Could you check a few things on this model? Use its own coordinates, in mm. A direction names the side the tool comes from. Round coordinates to 2 decimals unless told otherwise and drop trailing zeros. Write each loop counter-clockwise with the first axis right and the second up, starting at its lowest first coordinate (ties: lowest second). Pieces come first, ordered by that corner, then holes. Notation, with made-up numbers: (-17, 20) -> (24, 20) arc R31 ccw to (24, 49) -> close; hole circle Ø7 at (40.5, 59.25). An arc over 180 degrees is marked (long way). One line per question, with ' | ' between items. Start each with the question number.
1. If I drill on line 1 along Z through (x, y) = (-2.5, -3.5); line 2 along Z through (x, y) = (5, 1); line 3 along X through (y, z) = (-3.25, 11), over which ranges is the centre line in solid material (lowest first)? Write a range as [from, to].
2. For pin 1 Ø2 at (x, z) = (-4, 10.5) entering from +Y; pin 2 Ø2 at (x, z) = (5, 4.5) entering from +Y; pin 3 Ø2 at (y, z) = (-3, 8) entering from -X, each with a flat end and sliding along its axis, tell me the tip position at first contact or that it passes through.
3. For faces 1 (the flat face through (0, 0, 0)), 2 (the conical face through (-0.86, -3.87, 6.76)), which set-ups out of +Z, -Z, +X, -X, +Y, -Y let a thin tool reach every point of the face, with its end or its side?
4. Imagine slicing it at D-D, the plane z = 4.5. List the corners of the cut face in (x, y) for me.
5. Imagine slicing it at C-C, the plane z = 2. List the corners of the cut face in (x, y) for me.
Autodesk Inventor part; units mm, degrees
ref_plane "YZ Plane" through (0, 0, 0) normal (1, 0, 0) x (0, 1, 0)
ref_plane "XZ Plane" through (0, 0, 0) normal (0, 1, 0) x (-1, 0, 0)
ref_plane "XY Plane" through (0, 0, 0) normal (0, 0, 1) x (1, 0, 0)
sketch "Sketch1" plane through (0, 0, 0) normal (0, 0, 1) x (1, 0, 0)
  circle A0 centre (0, 0) radius 6.35
  dimension "d0" = 12.7
extrude "Extrusion1" add sketch "Sketch1" along normal blind 6.604
chamfer "Chamfer1" distance 2.54 angle 45 1 edges at (-6.35, 0, 6.604)
sketch "Sketch2" plane through (0, 0, 6.604) normal (0, 0, 1) x (1, 0, 0)
  circle A0 centre (0, 0) radius 6.35
  dimension "d6" = 12.7
extrude "Extrusion2" add sketch "Sketch2" along normal blind 6.604
chamfer "Chamfer2" distance 2.54 angle 45 1 edges at (-6.35, 0, 6.604)
properties part number "LiftPully" material "Aluminum 6061"
Geometry results:
1) line 1: z = [0, 6.11], [7.09, 13.21] | line 2: z = [0, 5.31], [7.89, 13.21] | line 3: x = [-5.46, 5.46]
2) pin 1: stops at y = 5.6 | pin 2: stops at y = 4.85 | pin 3: stops at x = -5.54
3) face 1: -Z, +X, -X, +Y, -Y | face 2: none
4) outline: circle Ø11.83 at (0, 0)
5) outline: circle Ø12.7 at (0, 0)
